from build123d import *

# Parameters (mm, degrees)
AXLE_BASE_SKETCH_R        = 26
AXLE_DEPTH                = 61.5
GUARD_BASE_R              = 37.5
GUARD_DEPTH               = 5
INNER_AXLE_HOLE_BASE_R    = 8.5
INNER_AXLE_HOLE_DEPTH     = 67.5
BEND_START                = -49.25
BEND_ROOM_BASE_W          = 1.5
BEND_ROOM_BASE_H          = 75
BEND_ROOM_1_DEPTH         = 49.25
BEND_ROOM_2_COUNT         = 2
BEND_ROOM_2_ANGLE         = 90
EASY_REMOVAL_CHAMFER_SIZE = 4


with BuildPart() as part:
    # Axle base sketch → Axle (new body)
    with BuildSketch(Plane.XY):
        Circle(AXLE_BASE_SKETCH_R)
    extrude(amount=AXLE_DEPTH)

    # Guard base → Guard (add)
    with BuildSketch(Plane(origin=(0, 0, 0), x_dir=(-1, 0, 0), z_dir=(0, 0, -1))):
        Circle(GUARD_BASE_R)
    extrude(amount=GUARD_DEPTH)

    # Inner axle hole base → Inner axle hole (cut, through all)
    with BuildSketch(Plane.XY.offset(61.5)):
        Circle(INNER_AXLE_HOLE_BASE_R)
    extrude(amount=-INNER_AXLE_HOLE_DEPTH, mode=Mode.SUBTRACT)

    # Mate ring base → Mate rings (revolve)
    with BuildSketch(Plane(origin=(0, 0, 0), x_dir=(1, 0, 0), z_dir=(0, 1, 0))):
        Polygon((26, -61.5), (26.75, -60.75), (26.75, -60), (26, -59.25), align=None)
        Polygon((26, -55.75), (26.75, -55), (26.75, -54.25), (26, -53.5), align=None)
    revolve(axis=Axis((0, 0, 0), (0, 0, -1)))

    # Inner mass remove base → Inner mass remove (revolve, cut)
    with BuildSketch(Plane(origin=(0, 0, 0), x_dir=(0, 0, -1), z_dir=(1, 0, 0))):
        Polygon((-61.5, 0), (-44.25, -17.25), (-12.25, -17.25), (5, 0), align=None)
    revolve(axis=Axis((0, 0, 0), (0, 0, -1)), mode=Mode.SUBTRACT)

    # Bend room base → Bend room 1 (cut)
    with BuildSketch(Plane.XY.offset(61.5).offset(BEND_START)):
        Rectangle(BEND_ROOM_BASE_W, BEND_ROOM_BASE_H)
    bend_room_1 = extrude(amount=BEND_ROOM_1_DEPTH, mode=Mode.SUBTRACT)

    # Bend room 2: Bend room 1 ×2 about axis
    bend_room_2_axis = Axis((0, 0, 0), (0, 0, -1))
    for i in range(1, BEND_ROOM_2_COUNT):
        add(bend_room_1.rotate(bend_room_2_axis, i * BEND_ROOM_2_ANGLE / (BEND_ROOM_2_COUNT - 1)), mode=Mode.SUBTRACT)

    # Easy removal chamfer
    easy_removal_chamfer_edges = [part.edges().sort_by_distance(p)[0] for p in [
        (37.5, 0, 0),
    ]]
    chamfer(easy_removal_chamfer_edges, length=EASY_REMOVAL_CHAMFER_SIZE)


solid = part.part
Could you check a few things on this model? Use its own coordinates, in mm. A direction names the side the tool comes from. Give positions to 0.01 mm unless a question says otherwise; leave off trailing zeros. Order: outer loops, then holes, each group sorted by start corner. A loop starts at its lowest first (then second) coordinate and runs counter-clockwise, first axis right, second up. Notation, with made-up numbers: (56.25, -39) - (96.25, -39) arc R7 ccw to (96.25, -32) - close; hole circle Ø4 at (59.25, 3.25). An arc over 180 degrees is marked (long way). Return JSON: item names as keys, results as strings. Group by question number.
Q1. Suppose I cut it at B-B, the plane z = 7.5. Please give me the cut outline in (x, y).
Q2. Please list where these lines run through material, in increasing order: line 1 along X through (y, z) = (0, 1); line 2 along Y through (x, z) = (-1, 15). Write a range as [from, to].
Q3. Thinking about a two-plate mould opening in Z: for faces 1 (the face through (-8.547, 8.372, 49.536)), 2 (the face through (-18.19, 18.58, 57.48)), 3 (the face through (-19.115, 18.713, 60.37)), which applies, pulls with the +Z half, pulls with the -Z half, needs draft (parallel to the pull), parting line crosses it, or undercut?
Q4. Suppose I cut it at A-A, the plane z = 19.5. Please give me the cut outline in (x, y), and give its area (3 significant figures).
Q5. Will these pins go through, and if not, where does the flat tip stop? pin 1 Ø20 at (x, z) = (-18, 42.5) entering from +Y; pin 2 Ø9 at (x, z) = (17, 45.5) entering from +Y; pin 3 Ø12 at (y, z) = (-19.5, 4) entering from -X.
Q6. Which directions (+Z, -Z, +X, -X, +Y, -Y) give clear straight access to the entire face, cutting with the end or side of a thin tool? Please do faces 4 (the face through (19.115, -18.713, 54.62)), 5 (the face through (-20, 0.75, 42)), 6 (the face through (18.58, 18.19, 57.48)), 7 (the face through (6.07, 5.95, 57.31)), 8 (the face through (12.07, 12.324, 28.026)).
Resolved:
{
 "1": {"outline": "circle Ø52 at (0, 0); hole circle Ø25 at (0, 0)"},
 "2": {"line 1": "x = [-26, -8.5], [8.5, 26]", "line 2": "y = [-25.98, -17.22], [17.22, 25.98]"},
 "3": {"face 1": "undercut", "face 2": "undercut", "face 3": "needs draft"},
 "4": {"outline": "(-25.99, -0.75) arc R26 ccw to (-0.75, -25.99) - (-0.75, -17.23) arc R17.25 cw to (-17.23, -0.75) - close; (-25.99, 0.75) - (-17.23, 0.75) arc R17.25 cw to (-0.75, 17.23) - (-0.75, 25.99) arc R26 ccw to start; (0.75, -25.99) arc R26 ccw to (25.99, -0.75) - (17.23, -0.75) arc R17.25 cw to (0.75, -17.23) - close; (0.75, 17.23) arc R17.25 cw to (17.23, 0.75) - (25.99, 0.75) arc R26 ccw to (0.75, 25.99) - close", "area": "1,140 mm2"},
 "5": {"pin 1": "stops at y = 24.74", "pin 2": "stops at y = 22.8", "pin 3": "stops at x = -30.54"},
 "6": {"face 4": "+Z, +X, -Y", "face 5": "+Z, +X, -X", "face 6": "+X, +Y", "face 7": "+Z, -Z", "face 8": "none"}
}
